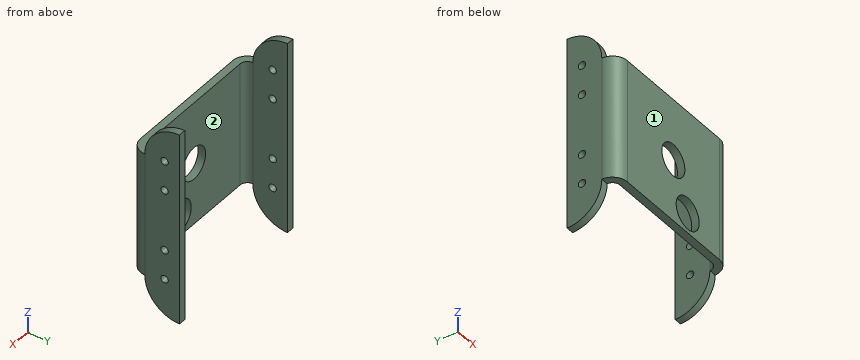
```python
from build123d import *

# Parameters (mm, degrees)
BASE_FLANGE1_DEPTH      = 156
CUT_EXTRUDE1_DEPTH      = 206.71825393
SKETCH6_R               = 13
CUT_EXTRUDE2_DEPTH      = 10
CUT_EXTRUDE3_DEPTH      = 203.039600079
CUT_EXTRUDE3_DEPTH_BACK = 203.039600079
SKETCH7_R               = 3


# Sheet-metal steps are written as plain solids
with BuildPart() as part:
    # Sketch2 → Base-Flange1 (new body)
    with BuildSketch(Plane.XY):
        with BuildLine():
            Line((-29.957142857, 40), (-29.957142857, 12))
            ThreePointArc((-29.957142857, 12), (-26.442424231, 3.514718626), (-17.957142857, 0))
            Line((-17.957142857, 0), (86.042857143, 0))
            ThreePointArc((86.042857143, 0), (94.528138517, 3.514718626), (98.042857143, 12))
            Line((98.042857143, 12), (98.042857143, 40))
            Line((98.042857143, 40), (92.042857143, 40))
            Line((92.042857143, 40), (92.042857143, 12))
            ThreePointArc((92.042857143, 12), (90.28549783, 7.757359313), (86.042857143, 6))
            Line((86.042857143, 6), (-17.957142857, 6))
            ThreePointArc((-17.957142857, 6), (-22.199783544, 7.757359313), (-23.957142857, 12))
            Line((-23.957142857, 12), (-23.957142857, 40))
            Line((-23.957142857, 40), (-29.957142857, 40))
        make_face()
    extrude(amount=BASE_FLANGE1_DEPTH)

    # Sketch5 → Cut-Extrude1 (cut, through all)
    with BuildSketch(Plane(origin=(98.042857143, 0, 0), x_dir=(0, 0, -1), z_dir=(1, 0, 0))):
        with BuildLine():
            Line((-128, 12), (-128, 0))
            Line((-128, 0), (-156, 0))
            Line((-156, 0), (-156, 40))
            ThreePointArc((-156, 40), (-147.798989873, 20.201010127), (-128, 12))
        make_face()
        with BuildLine():
            Line((0, 0), (0, 40))
            ThreePointArc((0, 40), (-8.201010127, 20.201010127), (-28, 12))
            Line((-28, 12), (-28, 0))
            Line((-28, 0), (0, 0))
        make_face()
    extrude(amount=-CUT_EXTRUDE1_DEPTH, mode=Mode.SUBTRACT)

    # Sketch6 → Cut-Extrude2 (cut)
    with BuildSketch(Plane.XZ):
        with Locations(Location((34.042857143, 78, 0), (0, 0, 270))):
            Circle(SKETCH6_R)
        with Locations(Location((50.212608526, 44, 0), (0, 0, 270))):
            Circle(SKETCH6_R)
    extrude(amount=-CUT_EXTRUDE2_DEPTH, mode=Mode.SUBTRACT)

    # Sketch7 → Cut-Extrude3 (cut, two sides: drawn at the far end of the back side and taken through both)
    with BuildSketch(Plane.ZY.offset(-92.042857143).offset(-CUT_EXTRUDE3_DEPTH_BACK)):
        with Locations((31.647353532, 28)):
            Circle(SKETCH7_R)
        with Locations((55.647353532, 28)):
            Circle(SKETCH7_R)
        with Locations((105, 28)):
            Circle(SKETCH7_R)
        with Locations((129, 28)):
            Circle(SKETCH7_R)
    extrude(amount=CUT_EXTRUDE3_DEPTH + CUT_EXTRUDE3_DEPTH_BACK, mode=Mode.SUBTRACT)


solid = part.part
```
Model file for the job. Use its own axes, mm. Face numbers are marked on the shaded views. A direction names the side the tool comes from. Round coordinates to 2 decimals unless told otherwise and drop trailing zeros. Write each loop counter-clockwise with the first axis right and the second up, starting at its lowest first coordinate (ties: lowest second). Pieces come first, ordered by that corner, then holes. Notation, with made-up numbers: (60, 7) - (112, 7) arc R31 cw to (112, 38) - close; hole circle Ø1 at (11.25, -37). An arc over 180 degrees is marked (long way). One line per item, written item: value.
(1) Cut at C-C, the plane x = 28.5. Give the cut face in (y, z), plus the area to 3 significant figures.
Values follow:
outline: (0, 28) - (6, 28) - (6, 66.24) - (0, 66.24) - close; (0, 89.76) - (6, 89.76) - (6, 128) - (0, 128) - close
area: 459 mm²
(2) Cut at A-A, the plane z = 105. Give the cut face in (x, y), plus the area to 3 significant figures.
Values follow:
outline: (-29.96, 12) arc R12 ccw to (-17.96, 0) - (86.04, 0) arc R12 ccw to (98.04, 12) - (98.04, 25) - (92.04, 25) - (92.04, 12) arc R6 cw to (86.04, 6) - (-17.96, 6) arc R6 cw to (-23.96, 12) - (-23.96, 25) - (-29.96, 25) - close; (-29.96, 31) - (-23.96, 31) - (-23.96, 40) - (-29.96, 40) - close; (92.04, 31) - (98.04, 31) - (98.04, 40) - (92.04, 40) - close
area: 1,060 mm²
(3) Cut at B-B, the plane z = 44. Give the cut face in (x, y).
Values follow:
outline: (-29.96, 12) arc R12 ccw to (-17.96, 0) - (37.21, 0) - (37.21, 6) - (-17.96, 6) arc R6 cw to (-23.96, 12) - (-23.96, 40) - (-29.96, 40) - close; (63.21, 0) - (86.04, 0) arc R12 ccw to (98.04, 12) - (98.04, 40) - (92.04, 40) - (92.04, 12) arc R6 cw to (86.04, 6) - (63.21, 6) - close
(4) Wall check: probe 1 along X at (y, z) = (38.5, 31); probe 2 along Z at (x, y) = (93.4, 28); probe 3 along Y at (x, z) = (56.5, 119). Give the ranges that are in metal, low to high.
Values follow:
probe 1: x = -29.96 to -23.96, 92.04 to 98.04
probe 2: z = 2.7 to 28.65, 34.65 to 52.65, 58.65 to 102, 108 to 126, 132 to 153.3
probe 3: y = 0 to 6
(5) Cut at D-D, the plane y = 36.5. Give the cut face in (x, z).
Values follow:
outline: (-29.96, 0.22) - (-23.96, 0.22) - (-23.96, 155.78) - (-29.96, 155.78) - close; (92.04, 0.22) - (98.04, 0.22) - (98.04, 155.78) - (92.04, 155.78) - close
(6) Drop flat-ended pins along their axis: P1, Ø5, axis at y = 28, z = 55.65, coming from the -X side; P2, Ø9.5, axis at y = 28, z = 129, coming from the +X side; P3, Ø3.5, axis at x = 35.5, y = 7, coming from the +Z side. Give the stop position or say it passes through.
Values follow:
P1: passes through
P2: stops at x = 98.04
P3: stops at z = 128
(7) 3-axis set-ups, long thin cutter, end or side, ignore diameter. For the marked faces 1 and 2: which of +Z, -Z, +X, -X, +Y, -Y reach the whole face in a straight line?
Values follow:
face 1: +Z, -Z, +X, -X, -Y
face 2: +Z, -Z, +Y
